Model file for the job. Use its own axes, mm. Face numbers are marked on the shaded views. A direction names the side the tool comes from. Coordinates: 2 decimals unless noted, no trailing zeros. Loops run counter-clockwise (first coordinate to the right, second up) from the corner with the lowest first, then second, coordinate; pieces in that order, holes last. Notation, with made-up numbers: (-23, 72.5) -> (5, 72.5) arc R25 cw to (5, 92.5) -> close; hole circle Ø7 at (2.5, 86.25). An arc over 180 degrees is marked (long way). Use one line per item in the form item = value.
Autodesk Inventor part; units mm, degrees
ref_plane "YZ Plane" through (0, 0, 0) normal (1, 0, 0) x (0, 1, 0)
ref_plane "XZ Plane" through (0, 0, 0) normal (0, 1, 0) x (-1, 0, 0)
ref_plane "XY Plane" through (0, 0, 0) normal (0, 0, 1) x (1, 0, 0)
sketch "Sketch1" plane through (0, 0, 0) normal (0, 0, 1) x (1, 0, 0)
  arc A0 (-17.7023, -49.8275) -> (-15.7023, -51.8275) centre (-15.7023, -49.8275) ccw
  line L0 (-15.7023, -51.8275) -> (30.2977, -51.8275)
  arc A1 (30.2977, -51.8275) -> (32.2977, -49.8275) centre (30.2977, -49.8275) ccw
  line L1 (32.2977, -49.8275) -> (32.2977, -3.8275)
  arc A2 (32.2977, -3.8275) -> (30.2977, -1.8275) centre (30.2977, -3.8275) ccw
  line L2 (30.2977, -1.8275) -> (-15.7023, -1.8275)
  arc A3 (-15.7023, -1.8275) -> (-17.7023, -3.8275) centre (-15.7023, -3.8275) ccw
  line L3 (-17.7023, -3.8275) -> (-17.7023, -49.8275)
  circle A4 centre (-15.7023, -3.8275) radius 1.5
  circle A5 centre (-10.7525, -8.7773) radius 1.5
  circle A6 centre (-10.7525, -44.8778) radius 1.5
  circle A7 centre (-15.7023, -49.8275) radius 1.5
  circle A8 centre (25.348, -44.8778) radius 1.5
  circle A9 centre (30.2977, -49.8275) radius 1.5
  circle A10 centre (25.348, -8.7773) radius 1.5
  circle A11 centre (30.2977, -3.8275) radius 1.5
  circle A12 centre (7.2977, -26.8275) radius 8.5
  line L4 (-27.7023, 8.1725) -> (42.2977, 8.1725)
  line L5 (42.2977, 8.1725) -> (42.2977, -61.8275)
  line L6 (42.2977, -61.8275) -> (-27.7023, -61.8275)
  line L7 (-27.7023, -61.8275) -> (-27.7023, 8.1725)
  line L8 (-27.7023, 8.1725) -> (42.2977, -61.8275) construction
  line L9 (42.2977, 8.1725) -> (-27.7023, -61.8275) construction
  line L10 (42.2977, 8.1725) -> (-27.7023, 8.1725)
  line L11 (-27.7023, 8.1725) -> (-27.7023, 78.1725)
  line L12 (-27.7023, 78.1725) -> (42.2977, 78.1725)
  line L13 (42.2977, 78.1725) -> (42.2977, 8.1725)
  line L14 (11.2977, 68.1725) -> (38.2977, 68.1725)
  line L15 (38.2977, 68.1725) -> (38.2977, 18.1725)
  line L16 (38.2977, 18.1725) -> (11.2977, 18.1725)
  line L17 (11.2977, 18.1725) -> (11.2977, 68.1725)
  line L18 (11.2977, 68.1725) -> (38.2977, 18.1725) construction
  line L19 (38.2977, 68.1725) -> (11.2977, 18.1725) construction
  line L20 (-23.7023, 18.1725) -> (3.2977, 18.1725)
  line L21 (3.2977, 18.1725) -> (3.2977, 68.1725)
  line L22 (3.2977, 68.1725) -> (-23.7023, 68.1725)
  line L23 (-23.7023, 68.1725) -> (-23.7023, 18.1725)
  line L24 (-23.7023, 18.1725) -> (3.2977, 68.1725) construction
  line L25 (3.2977, 18.1725) -> (-23.7023, 68.1725) construction
  line L26 (4.7977, 69.6725) -> (4.7977, 16.6725)
  line L27 (-25.2023, 16.6725) -> (-25.2023, 69.6725)
  line L28 (-25.2023, 69.6725) -> (4.7977, 16.6725) construction
  line L29 (4.7977, 69.6725) -> (-25.2023, 16.6725) construction
  line L30 (39.7977, 69.6725) -> (39.7977, 16.6725)
  line L31 (9.7977, 16.6725) -> (9.7977, 69.6725)
  line L32 (9.7977, 69.6725) -> (39.7977, 16.6725) construction
  line L33 (39.7977, 69.6725) -> (9.7977, 16.6725) construction
  line L34 (38.2977, 68.1725) -> (38.2977, 69.6725)
  line L35 (11.2977, 68.1725) -> (11.2977, 69.6725)
  line L36 (11.2977, 18.1725) -> (11.2977, 16.6725)
  line L37 (38.2977, 18.1725) -> (38.2977, 16.6725)
  line L38 (3.2977, 69.6725) -> (3.2977, 68.1725)
  line L39 (3.2977, 18.1725) -> (3.2977, 16.6725)
  line L40 (-23.7023, 68.1725) -> (-23.7023, 69.6725)
  line L41 (-23.7023, 18.1725) -> (-23.7023, 16.6725)
  line L42 (-25.2023, 69.6725) -> (-23.7023, 69.6725)
  line L43 (3.2977, 69.6725) -> (4.7977, 69.6725)
  line L44 (4.7977, 16.6725) -> (3.2977, 16.6725)
  line L45 (-23.7023, 16.6725) -> (-25.2023, 16.6725)
  line L46 (39.7977, 16.6725) -> (38.2977, 16.6725)
  line L47 (11.2977, 16.6725) -> (9.7977, 16.6725)
  line L48 (9.7977, 69.6725) -> (11.2977, 69.6725)
  line L49 (38.2977, 69.6725) -> (39.7977, 69.6725)
  point P0 (0, 0)
  point P1 (24.7977, 43.1725)
  point P2 (-10.2023, 43.1725)
  dimension "d0" = 70
  dimension "d1" = 70
  dimension "d2" = 70
  dimension "d3" = 27
  dimension "d4" = 50
  dimension "d5" = 27
  dimension "d6" = 30
  dimension "d7" = 53
  dimension "d8" = 30
  dimension "d9" = 53
sketch "Sketch2" plane through (0, 0, 0) normal (0, 0, 1) x (1, 0, 0)
  arc A0 (-17.7023, -49.8275) -> (-15.7023, -51.8275) centre (-15.7023, -49.8275) ccw
  line L0 (-15.7023, -51.8275) -> (30.2977, -51.8275)
  arc A1 (30.2977, -51.8275) -> (32.2977, -49.8275) centre (30.2977, -49.8275) ccw
  line L1 (32.2977, -49.8275) -> (32.2977, -3.8275)
  arc A2 (32.2977, -3.8275) -> (30.2977, -1.8275) centre (30.2977, -3.8275) ccw
  line L2 (30.2977, -1.8275) -> (-15.7023, -1.8275)
  arc A3 (-15.7023, -1.8275) -> (-17.7023, -3.8275) centre (-15.7023, -3.8275) ccw
  line L3 (-17.7023, -3.8275) -> (-17.7023, -49.8275)
  circle A4 centre (-15.7023, -3.8275) radius 1.5
  circle A5 centre (-10.7525, -8.7773) radius 1.5
  circle A6 centre (-10.7525, -44.8778) radius 1.5
  circle A7 centre (-15.7023, -49.8275) radius 1.5
  circle A8 centre (25.348, -44.8778) radius 1.5
  circle A9 centre (30.2977, -49.8275) radius 1.5
  circle A10 centre (25.348, -8.7773) radius 1.5
  circle A11 centre (30.2977, -3.8275) radius 1.5
  circle A12 centre (7.2977, -26.8275) radius 8.5
  line L4 (-27.7023, 18.1725) -> (42.2977, 18.1725)
  line L5 (42.2977, 18.1725) -> (42.2977, -61.8275)
  line L6 (42.2977, -61.8275) -> (-27.7023, -61.8275)
  line L7 (-27.7023, -61.8275) -> (-27.7023, 18.1725)
  line L8 (42.2977, 18.1725) -> (-27.7023, 18.1725)
  line L9 (-27.7023, 18.1725) -> (-27.7023, 88.1725)
  line L10 (-27.7023, 88.1725) -> (42.2977, 88.1725)
  line L11 (42.2977, 88.1725) -> (42.2977, 18.1725)
  line L12 (11.2977, 78.1725) -> (38.2977, 78.1725)
  line L13 (38.2977, 78.1725) -> (38.2977, 28.1725)
  line L14 (38.2977, 28.1725) -> (11.2977, 28.1725)
  line L15 (11.2977, 28.1725) -> (11.2977, 78.1725)
  line L16 (11.2977, 78.1725) -> (38.2977, 28.1725) construction
  line L17 (38.2977, 78.1725) -> (11.2977, 28.1725) construction
  line L18 (-23.7023, 28.1725) -> (3.2977, 28.1725)
  line L19 (3.2977, 28.1725) -> (3.2977, 78.1725)
  line L20 (3.2977, 78.1725) -> (-23.7023, 78.1725)
  line L21 (-23.7023, 78.1725) -> (-23.7023, 28.1725)
  line L22 (-23.7023, 28.1725) -> (3.2977, 78.1725) construction
  line L23 (3.2977, 28.1725) -> (-23.7023, 78.1725) construction
  line L24 (4.7977, 79.6725) -> (4.7977, 26.6725)
  line L25 (-25.2023, 26.6725) -> (-25.2023, 79.6725)
  line L26 (-25.2023, 79.6725) -> (4.7977, 26.6725) construction
  line L27 (4.7977, 79.6725) -> (-25.2023, 26.6725) construction
  line L28 (39.7977, 79.6725) -> (39.7977, 26.6725)
  line L29 (9.7977, 26.6725) -> (9.7977, 79.6725)
  line L30 (9.7977, 79.6725) -> (39.7977, 26.6725) construction
  line L31 (39.7977, 79.6725) -> (9.7977, 26.6725) construction
  line L32 (38.2977, 78.1725) -> (38.2977, 79.6725)
  line L33 (11.2977, 78.1725) -> (11.2977, 79.6725)
  line L34 (11.2977, 28.1725) -> (11.2977, 26.6725)
  line L35 (38.2977, 28.1725) -> (38.2977, 26.6725)
  line L36 (3.2977, 79.6725) -> (3.2977, 78.1725)
  line L37 (3.2977, 28.1725) -> (3.2977, 26.6725)
  line L38 (-23.7023, 78.1725) -> (-23.7023, 79.6725)
  line L39 (-23.7023, 28.1725) -> (-23.7023, 26.6725)
  line L40 (-25.2023, 79.6725) -> (-23.7023, 79.6725)
  line L41 (3.2977, 79.6725) -> (4.7977, 79.6725)
  line L42 (4.7977, 26.6725) -> (3.2977, 26.6725)
  line L43 (-23.7023, 26.6725) -> (-25.2023, 26.6725)
  line L44 (39.7977, 26.6725) -> (38.2977, 26.6725)
  line L45 (11.2977, 26.6725) -> (9.7977, 26.6725)
  line L46 (9.7977, 79.6725) -> (11.2977, 79.6725)
  line L47 (38.2977, 79.6725) -> (39.7977, 79.6725)
  point P0 (0, 0)
  point P1 (0, 0)
  point P2 (24.7977, 53.1725)
  point P3 (-10.2023, 53.1725)
  dimension "d10" = 70
  dimension "d11" = 80
  dimension "d13" = 27
  dimension "d14" = 50
  dimension "d15" = 27
  dimension "d16" = 30
  dimension "d17" = 53
  dimension "d18" = 30
  dimension "d19" = 53
  dimension "d52" = 10
  dimension "d53" = 10
  dimension "d55" = 10
extrude "Extrusion1" add sketch "Sketch1" against normal blind 3 contours L3 A3 L2 A2 L1 A1 L0 A0 | A4 | A5 | A6 | A7 | A8 | A9 | A10 | A11 | A12 | L11 L12 L13 L4 | L4 L5 L6 L7 | L14 L15 L16 L17 | L17 L36 L47 L31 L48 L35 | L34 L49 L30 L46 L37 L15 | L23 L22 L21 L20 | L41 L45 L27 L42 L40 L23 | L21 L38 L43 L26 L44 L39
extrude "Extrusion2" add sketch "Sketch2" along normal blind 8 contours L15 L34 L45 L29 L46 L33 | L32 L47 L28 L44 L35 L13 | L39 L43 L25 L40 L38 L21 | L19 L36 L41 L24 L42 L37
sketch "Sketch3" plane through (0, 0, 0) normal (0, 0, 1) x (1, 0, 0)
  arc A0 (-17.7023, -49.8275) -> (-15.7023, -51.8275) centre (-15.7023, -49.8275) ccw
  line L0 (-15.7023, -51.8275) -> (30.2977, -51.8275)
  arc A1 (30.2977, -51.8275) -> (32.2977, -49.8275) centre (30.2977, -49.8275) ccw
  line L1 (32.2977, -49.8275) -> (32.2977, -3.8275)
  arc A2 (32.2977, -3.8275) -> (30.2977, -1.8275) centre (30.2977, -3.8275) ccw
  line L2 (30.2977, -1.8275) -> (-15.7023, -1.8275)
  arc A3 (-15.7023, -1.8275) -> (-17.7023, -3.8275) centre (-15.7023, -3.8275) ccw
  line L3 (-17.7023, -3.8275) -> (-17.7023, -49.8275)
  circle A4 centre (-15.7023, -3.8275) radius 1.5
  circle A5 centre (-10.7525, -8.7773) radius 1.5
  circle A6 centre (-10.7525, -44.8778) radius 1.5
  circle A7 centre (-15.7023, -49.8275) radius 1.5
  circle A8 centre (25.348, -44.8778) radius 1.5
  circle A9 centre (30.2977, -49.8275) radius 1.5
  circle A10 centre (25.348, -8.7773) radius 1.5
  circle A11 centre (30.2977, -3.8275) radius 1.5
  circle A12 centre (7.2977, -26.8275) radius 8.5
  line L4 (-27.7023, 8.1725) -> (42.2977, 8.1725)
  line L5 (42.2977, 8.1725) -> (42.2977, -61.8275)
  line L6 (42.2977, -61.8275) -> (-27.7023, -61.8275)
  line L7 (-27.7023, -61.8275) -> (-27.7023, 8.1725)
  line L8 (-27.7023, 8.1725) -> (42.2977, -61.8275) construction
  line L9 (42.2977, 8.1725) -> (-27.7023, -61.8275) construction
  line L10 (42.2977, 8.1725) -> (-27.7023, 8.1725)
  line L11 (-27.7023, 8.1725) -> (-27.7023, 78.1725)
  line L12 (-27.7023, 78.1725) -> (42.2977, 78.1725)
  line L13 (42.2977, 78.1725) -> (42.2977, 8.1725)
  line L14 (11.2977, 68.1725) -> (38.2977, 68.1725)
  line L15 (38.2977, 68.1725) -> (38.2977, 18.1725)
  line L16 (38.2977, 18.1725) -> (11.2977, 18.1725)
  line L17 (11.2977, 18.1725) -> (11.2977, 68.1725)
  line L18 (11.2977, 68.1725) -> (38.2977, 18.1725) construction
  line L19 (38.2977, 68.1725) -> (11.2977, 18.1725) construction
  line L20 (-23.7023, 18.1725) -> (3.2977, 18.1725)
  line L21 (3.2977, 18.1725) -> (3.2977, 68.1725)
  line L22 (3.2977, 68.1725) -> (-23.7023, 68.1725)
  line L23 (-23.7023, 68.1725) -> (-23.7023, 18.1725)
  line L24 (-23.7023, 18.1725) -> (3.2977, 68.1725) construction
  line L25 (3.2977, 18.1725) -> (-23.7023, 68.1725) construction
  line L26 (4.7977, 69.6725) -> (4.7977, 16.6725)
  line L27 (-25.2023, 16.6725) -> (-25.2023, 69.6725)
  line L28 (-25.2023, 69.6725) -> (4.7977, 16.6725) construction
  line L29 (4.7977, 69.6725) -> (-25.2023, 16.6725) construction
  line L30 (39.7977, 69.6725) -> (39.7977, 16.6725)
  line L31 (9.7977, 16.6725) -> (9.7977, 69.6725)
  line L32 (9.7977, 69.6725) -> (39.7977, 16.6725) construction
  line L33 (39.7977, 69.6725) -> (9.7977, 16.6725) construction
  line L34 (38.2977, 68.1725) -> (38.2977, 69.6725)
  line L35 (11.2977, 68.1725) -> (11.2977, 69.6725)
  line L36 (11.2977, 18.1725) -> (11.2977, 16.6725)
  line L37 (38.2977, 18.1725) -> (38.2977, 16.6725)
  line L38 (3.2977, 69.6725) -> (3.2977, 68.1725)
  line L39 (3.2977, 18.1725) -> (3.2977, 16.6725)
  line L40 (-23.7023, 68.1725) -> (-23.7023, 69.6725)
  line L41 (-23.7023, 18.1725) -> (-23.7023, 16.6725)
  line L42 (-25.2023, 69.6725) -> (-23.7023, 69.6725)
  line L43 (3.2977, 69.6725) -> (4.7977, 69.6725)
  line L44 (4.7977, 16.6725) -> (3.2977, 16.6725)
  line L45 (-23.7023, 16.6725) -> (-25.2023, 16.6725)
  line L46 (39.7977, 16.6725) -> (38.2977, 16.6725)
  line L47 (11.2977, 16.6725) -> (9.7977, 16.6725)
  line L48 (9.7977, 69.6725) -> (11.2977, 69.6725)
  line L49 (38.2977, 69.6725) -> (39.7977, 69.6725)
  point P0 (0, 0)
  point P1 (0, 0)
  point P2 (0, 0)
  point P3 (24.7977, 43.1725)
  point P4 (-10.2023, 43.1725)
  dimension "d24" = 70
  dimension "d25" = 70
  dimension "d26" = 70
  dimension "d27" = 27
  dimension "d28" = 50
  dimension "d29" = 27
  dimension "d30" = 30
  dimension "d31" = 53
  dimension "d32" = 30
  dimension "d33" = 53
extrude "Extrusion3" add sketch "Sketch3" along normal blind 10 contours A12
sketch "Sketch4" plane through (0, 0, 0) normal (0, 0, 1) x (1, 0, 0)
  line L0 (-27.7023, 78.1725) -> (-27.7023, -61.8275)
  line L1 (-27.7023, -61.8275) -> (-22.7023, -61.8275)
  line L2 (-22.7023, -61.8275) -> (-22.7023, -46.8275)
  line L3 (-22.7023, -46.8275) -> (-27.7023, -46.8275)
  line L4 (-27.7023, -46.8275) -> (-27.7023, -61.8275)
  line L5 (42.3055, -61.8275) -> (37.3055, -61.8275)
  line L6 (37.3055, -61.8275) -> (37.3055, -46.8275)
  line L7 (37.3055, -46.8275) -> (42.3055, -46.8275)
  line L8 (42.3055, -46.8275) -> (42.3055, -61.8275)
  point P0 (0, 0)
  dimension "d36" = 5
  dimension "d37" = 15
  dimension "d38" = 5
  dimension "d39" = 15
extrude "Extrusion4" cut sketch "Sketch4" against normal blind 3
sketch "Sketch5" plane through (-22.7023, -61.8275, 0) normal (-1, 0, 0) x (0, 0, 1)
  circle A0 centre (-1.5, 1.5) radius 1
  point P0 (0, 61.8275)
  point P1 (0, 0)
  dimension "d43" = 2
extrude "Extrusion5" add sketch "Sketch5" along normal up to surface (5 mm away)
sketch "Sketch6" plane through (37.3055, -61.8275, 0) normal (1, 0, 0) x (0, 0, -1)
  circle A0 centre (1.5, 1.5) radius 1
  point P0 (0, 61.8275)
  dimension "d46" = 2
extrude "Extrusion6" add sketch "Sketch6" along normal blind 5
properties part number "base_1"
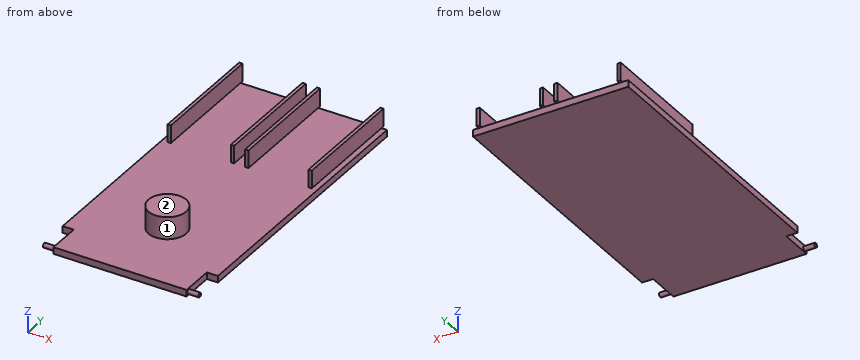
Q1. Which spindle directions (+Z, -Z, +X, -X, +Y, -Y) get a long thin tool onto all of the face, cutting with end or side? Do the marked faces 1 and 2. Say none if no direction does.
Result:
face_1 = +Z
face_2 = +Z, +X, -X, +Y, -Y
Q2. Band-saw the part on C-C, the plane y = -41.5. Write the cut outline in (x, z).
Result:
outline = (-27.7, -3) -> (42.3, -3) -> (42.3, 0) -> (-27.7, 0) -> close
Q3. Pin check, flat tips, straight feed: pin 1 Ø0.9 at (x, z) = (15.5, -1) entering from +Y; pin 2 Ø1.6 at (x, y) = (-24, 41) entering from +Z; pin 3 Ø1.5 at (x, z) = (-15, 2.5) entering from -Y; pin 4 Ø0.8 at (x, y) = (3.5, 79) entering from -Z. Stop position of each tip, or through.
Result:
pin_1 = 78.17
pin_2 = 8
pin_3 = through
pin_4 = 0
Q4. Band-saw the part on D-D, the plane x = 8. Write the cut outline in (y, z), and give its area (3 significant figures).
Result:
outline = (-61.83, -3) -> (78.17, -3) -> (78.17, 0) -> (-18.36, 0) -> (-18.36, 10) -> (-35.3, 10) -> (-35.3, 0) -> (-61.83, 0) -> close
area = 589 mm2
Q5. Wall check: line 1 along X through (y, z) = (39, 6); line 2 along Y through (x, z) = (27, -2); line 3 along X through (y, z) = (62, -1.5). Give the ranges that are in metal, low to high.
Result:
line_1 = -25.2 to -23.7, 3.3 to 4.8, 9.8 to 11.3, 38.3 to 39.8
line_2 = -61.83 to 78.17
line_3 = -27.7 to 42.3
Q6. Band-saw the part on A-A, the plane z = 3.25. Write the cut outline in (x, y).
Result:
outline = (-25.2, 26.67) -> (-23.7, 26.67) -> (-23.7, 79.67) -> (-25.2, 79.67) -> close; circle Ø17 at (7.3, -26.83); (3.3, 26.67) -> (4.8, 26.67) -> (4.8, 79.67) -> (3.3, 79.67) -> close; (9.8, 26.67) -> (11.3, 26.67) -> (11.3, 79.67) -> (9.8, 79.67) -> close; (38.3, 26.67) -> (39.8, 26.67) -> (39.8, 79.67) -> (38.3, 79.67) -> close
Q7. Band-saw the part on B-B, the plane x = 18. Write the cut outline in (y, z), and give its area (3 significant figures).
Result:
outline = (-61.83, -3) -> (78.17, -3) -> (78.17, 0) -> (-61.83, 0) -> close
area = 420 mm2
